Design review of the part built by this model. Coordinates are the model's own, in mm. A direction names the side the tool comes from. Round coordinates to 2 decimals unless told otherwise and drop trailing zeros. Loops run counter-clockwise (first coordinate to the right, second up) from the corner with the lowest first, then second, coordinate; pieces in that order, holes last. Notation, with made-up numbers: (50, 88.5) -> (96, 88.5) arc R24 cw to (96, 107.5) -> close; hole circle Ø8 at (62.5, 28). An arc over 180 degrees is marked (long way). Answer as CSV lines item,"result". Start each with the question number.
```python
from build123d import *

# Parameters (mm, degrees)
BOSS_EXTRUDE1_DEPTH = 10
SKETCH2_R           = 32.6
BOSS_EXTRUDE2_DEPTH = 1.5
CUT_EXTRUDE1_START  = -10
SKETCH3_R           = 32.6
SKETCH3_R_2         = 22.5
CUT_EXTRUDE1_DEPTH  = 8
SKETCH6_R           = 1.6
CUT_EXTRUDE4_DEPTH  = 10
SKETCH7_R           = 8.55
CUT_EXTRUDE5_DEPTH  = 7.5
SKETCH5_R           = 49.2
SKETCH5_R_2         = 41
CUT_EXTRUDE7_DEPTH  = 6
SKETCH9_R           = 1.6
CUT_EXTRUDE8_DEPTH  = 139.702018731
SKETCH10_R          = 22.55
CUT_EXTRUDE9_DEPTH  = 139.702018731
CUT_EXTRUDE10_DEPTH = 139.702018731


with BuildPart() as part:
    # Sketch1 → Boss-Extrude1 (new body)
    with BuildSketch(Plane.XY):
        with BuildLine():
            Line((-125, 59), (0, 59))
            ThreePointArc((0, 59), (59, 0), (0, -59))
            Line((0, -59), (-125, -59))
            Line((-125, -59), (-125, 59))
        make_face()
    extrude(amount=BOSS_EXTRUDE1_DEPTH)

    # Sketch2 → Boss-Extrude2 (add)
    with BuildSketch(Plane.XY.offset(10)):
        Circle(SKETCH2_R)
    extrude(amount=BOSS_EXTRUDE2_DEPTH)

    # Sketch3 → Cut-Extrude1 (cut)
    with BuildSketch(Plane.XY.offset(10).offset(CUT_EXTRUDE1_START)):
        Circle(SKETCH3_R)
        Circle(SKETCH3_R_2, mode=Mode.SUBTRACT)
    extrude(amount=CUT_EXTRUDE1_DEPTH, mode=Mode.SUBTRACT)

    # Sketch6 → Cut-Extrude4 (cut)
    with BuildSketch(Plane.XY.offset(10)):
        with Locations((0, -55)):
            Circle(SKETCH6_R)
        with Locations((-110, -55)):
            Circle(SKETCH6_R)
        with Locations((-110, 55)):
            Circle(SKETCH6_R)
        with Locations((0, 55)):
            Circle(SKETCH6_R)
    extrude(amount=-CUT_EXTRUDE4_DEPTH, mode=Mode.SUBTRACT)

    # Sketch7 → Cut-Extrude5 (cut)
    with BuildSketch(Plane(origin=(0, 0, 0), x_dir=(-1, 0, 0), z_dir=(0, 0, -1))):
        with Locations((95, 0)):
            Circle(SKETCH7_R)
    extrude(amount=-CUT_EXTRUDE5_DEPTH, mode=Mode.SUBTRACT)

    # Sketch5 → Cut-Extrude7 (cut)
    with BuildSketch(Plane.XY.offset(10)):
        Circle(SKETCH5_R)
        Circle(SKETCH5_R_2, mode=Mode.SUBTRACT)
    extrude(amount=-CUT_EXTRUDE7_DEPTH, mode=Mode.SUBTRACT)

    # Sketch9 → Cut-Extrude8 (cut, through all)
    with BuildSketch(Plane(origin=(0, 0, 0), x_dir=(-1, 0, 0), z_dir=(0, 0, -1))):
        with Locations((79.5, -15.5)):
            Circle(SKETCH9_R)
        with Locations((79.5, 15.5)):
            Circle(SKETCH9_R)
        with Locations((110.5, 15.5)):
            Circle(SKETCH9_R)
        with Locations((110.5, -15.5)):
            Circle(SKETCH9_R)
    extrude(amount=-CUT_EXTRUDE8_DEPTH, mode=Mode.SUBTRACT)

    # Sketch10 → Cut-Extrude9 (cut, through all)
    with BuildSketch(Plane(origin=(0, 0, 0), x_dir=(-1, 0, 0), z_dir=(0, 0, -1))):
        Circle(SKETCH10_R)
    extrude(amount=-CUT_EXTRUDE9_DEPTH, mode=Mode.SUBTRACT)

    # Sketch11 → Cut-Extrude10 (cut, through all)
    with BuildSketch(Plane(origin=(0, 0, 0), x_dir=(-1, 0, 0), z_dir=(0, 0, -1))):
        with BuildLine():
            Line((65, -24), (65, -11))
            ThreePointArc((65, -11), (64.707106781, -10.292893219), (64, -10))
            Line((64, -10), (62.8, -10))
            ThreePointArc((62.8, -10), (62.092893219, -10.292893219), (61.8, -11))
            Line((61.8, -11), (61.8, -24))
            ThreePointArc((61.8, -24), (62.092893219, -24.707106781), (62.8, -25))
            Line((62.8, -25), (64, -25))
            ThreePointArc((64, -25), (64.707106781, -24.707106781), (65, -24))
        make_face()
        with BuildLine():
            Line((62.8, 25), (64, 25))
            ThreePointArc((64, 25), (64.707106781, 24.707106781), (65, 24))
            Line((65, 24), (65, 11))
            ThreePointArc((65, 11), (64.707106781, 10.292893219), (64, 10))
            Line((64, 10), (62.8, 10))
            ThreePointArc((62.8, 10), (62.092893219, 10.292893219), (61.8, 11))
            Line((61.8, 11), (61.8, 24))
            ThreePointArc((61.8, 24), (62.092893219, 24.707106781), (62.8, 25))
        make_face()
    extrude(amount=-CUT_EXTRUDE10_DEPTH, mode=Mode.SUBTRACT)


solid = part.part
```
Q1. Add section B-B, the plane x = 20.5. Give the boundary of the cut face in (y, z).
Q2. Add section C-C, the plane y = -44.5. Give the boundary of the cut face in (x, z).
Q3. For pin 1 Ø3 at (y, z) = (19, 5.5) entering from +X; pin 2 Ø6 at (y, z) = (34, 7.5) entering from +X; pin 3 Ø4 at (x, y) = (-18, 29.5) entering from -Z; pin 4 Ø3.5 at (x, y) = (-79.5, 15.5) entering from +Z, all flat-tipped, find the tip position at first contact; note any pin that passes through.
Q4. Add section D-D, the plane x = -95. Give the boundary of the cut face in (y, z).
Q5. Mouldability with a two-part tool opening along X and no side actions: class faces 5 (the cylindrical face through (-25.9, -19.8, 10.7)), 6 (the flat face through (-52, 1, 10)), 7 (the flat face through (-65, -18, 5)) as pulls with the +X half, pulls with the -X half, needs draft (parallel to the pull), parting line crosses it, or undercut.
Q6. To check wall thickness, follow probe 1 along X at (y, z) = (0.5, 8.5); probe 2 along Y at (x, z) = (-110, 5.5); probe 3 along Y at (x, z) = (-110.5, 7). State the ranges of each line that lie inside material, in increasing order. Write a range as from..to.
Q7. Machinability: for faces 1 (the flat face through (28, -18, 10)), 2 (the flat face through (-62, -59, 5)), 3 (the flat face through (-95, 0, 7.5)), 4 (the flat face through (-61.8, -17, 5)), which of the approach directions +Z, -Z, +X, -X, +Y, -Y give a long, thin tool a straight path to every point of the face, cutting with its end or side? Answer none if there is none.
Q8. Add section A-A, the plane z = 2.25. State how many separate pieces and enclosed holes the cut face has, and give its area (3 significant figures).
Worked answers:
1,outline,"(-55.32, 0) -> (-25.35, 0) -> (-25.35, 8) -> (-9.39, 8) -> (-9.39, 11.5) -> (-25.35, 11.5) -> (-25.35, 10) -> (-35.51, 10) -> (-35.51, 4) -> (-44.73, 4) -> (-44.73, 10) -> (-55.32, 10) -> close; (9.39, 8) -> (25.35, 8) -> (25.35, 0) -> (55.32, 0) -> (55.32, 10) -> (44.73, 10) -> (44.73, 4) -> (35.51, 4) -> (35.51, 10) -> (25.35, 10) -> (25.35, 11.5) -> (9.39, 11.5) -> close"
2,outline,"(-125, 0) -> (38.74, 0) -> (38.74, 10) -> (20.99, 10) -> (20.99, 4) -> (-20.99, 4) -> (-20.99, 10) -> (-125, 10) -> close"
3,pin 1,"stops at x = 56.34"
3,pin 2,"stops at x = 50.2"
3,pin 3,"stops at z = 0"
3,pin 4,"stops at z = 10"
4,outline,"(-59, 0) -> (-8.55, 0) -> (-8.55, 7.5) -> (8.55, 7.5) -> (8.55, 0) -> (59, 0) -> (59, 10) -> (-59, 10) -> close"
5,face 5,"parting line crosses it"
5,face 6,"needs draft"
5,face 7,"undercut"
6,probe 1,"x = -125..-49.2, -41..-22.54, 22.54..41, 49.2..59"
6,probe 2,"y = -59..-56.6, -53.4..-17.02, -13.98..13.98, 17.02..53.4, 56.6..59"
6,probe 3,"y = -59..-56.52, -53.48..-17.1, -13.9..13.9, 17.1..53.48, 56.52..59"
7,face 1,"+Z"
7,face 2,"+Z, -Z, +X, -X, -Y"
7,face 3,"-Z"
7,face 4,"+Z, -Z"
8,separate pieces,"1"
8,enclosed holes,"12"
8,area,"16,500 mm^2"
